Model file for the job. Use its own axes, mm. A direction names the side the tool comes from. Give positions to 0.01 mm unless a question says otherwise; leave off trailing zeros. Write each loop counter-clockwise with the first axis right and the second up, starting at its lowest first coordinate (ties: lowest second). Pieces come first, ordered by that corner, then holes. Notation, with made-up numbers: (77, 40) - (87, 40) arc R4 cw to (87, 47) - close; hole circle Ø5 at (-8, -29.75). An arc over 180 degrees is marked (long way). One line per item, written item: value. Start each with the question number.
(1) Cut at C-C, the plane y = 2.15. State how many separate pieces and enclosed holes the cut face has, and give its area (3 significant figures).
(2) Cut at A-A, the plane x = -10.5. List the corners of the cut face in (y, z).
(3) Cut at B-B, the plane z = -15. List the corners of the cut face in (x, y) (3 decimals), and give its area (3 significant figures).
(4) Probe L1, parallel to Z at x = 30, y = 1.95; L2, parallel to X at y = 2.25, z = 0 (3 decimals); L3, parallel to Z at x = -69, y = 3. List the from-to ranges inside material, lowest first.
(5) Drop flat-ended pins along their axis: P1, Ø2.5, axis at y = 3, z = -113.5, coming from the -X side; P2, Ø2.5, axis at x = 84.63, z = 48.25, coming from the +Y side. Give the stop position or say it passes through.
(6) 3-axis set-ups, long thin cutter, end or side, ignore diameter. For faces 1 (the face through (-19.95, 2.58, 82.46)), 2 (the face through (-119.76, 2.58, 119.36)): which of +Z, -Z, +X, -X, +Y, -Y reach the whole face in a straight line?
(7) Mould opens along Z. For faces 3 (the face through (54.03, 2.58, -94.58)), 4 (the face through (-119.76, 2.58, -119.36)), 5 (the face through (119.36, 2.58, 119.76)) say: pulls with the +Z half, pulls with the -Z half, needs draft (parallel to the pull), parting line crosses it, or undercut.
from build123d import *

# Parameters (mm, degrees)
SKETCH1_W               = 254
SKETCH1_H               = 254
PLATFORM_BASE_DEPTH     = 5.08
SKETCH5_W               = 97.79
SKETCH5_H               = 152.4
CUT_EXTRUDE3_DEPTH      = 180.676950108
SKETCH6_W               = 25.4
SKETCH6_H               = 5.08
CUT_EXTRUDE4_DEPTH      = 180.676950108
CORNER_ROUNDING_R       = 25.4
MIRROR6_COPY_1_SKETCH_W = 25.4
MIRROR6_COPY_1_SKETCH_H = 5.08
MIRROR6_COPY_1_DEPTH    = 180.676950108
SKETCH7_R               = 3.175
CUT_EXTRUDE5_DEPTH      = 180.676950108
SKETCH11_W              = 12.7
SKETCH11_H              = 5.08
CUT_EXTRUDE8_DEPTH      = 180.676950108
SKETCH12_W              = 19.05
SKETCH12_H              = 5.08
CUT_EXTRUDE10_DEPTH     = 16.51
SKETCH14_W              = 152.4
SKETCH14_H              = 8.030698274
CUT_EXTRUDE12_DEPTH     = 19.05
SKETCH16_W              = 76.2
SKETCH16_H              = 5.08
CUT_EXTRUDE14_DEPTH     = 44.45
CUT_EXTRUDE16_DEPTH     = 180.676950108
CUT_EXTRUDE18_DEPTH     = 180.676950108
CUT_EXTRUDE19_DEPTH     = 180.676950108
CUT_EXTRUDE20_DEPTH     = 180.676950108
SKETCH27_W              = 10.16
SKETCH27_H              = 5.08
BOSS_EXTRUDE1_DEPTH     = 177.8
SKETCH28_R              = 1.6
CUT_EXTRUDE22_DEPTH     = 180.676950108
SKETCH29_R              = 1.651
CUT_EXTRUDE23_DEPTH     = 180.676950108
SKETCH30_R              = 1.651
CUT_EXTRUDE24_DEPTH     = 180.676950108
SKETCH32_R              = 1.651
CUT_EXTRUDE26_DEPTH     = 180.676950108


with BuildPart() as part:
    # Sketch1 → Platform-Base (new body)
    with BuildSketch(Plane(origin=(0, 0, 0), x_dir=(1, 0, 0), z_dir=(0, 1, 0))):
        Rectangle(SKETCH1_W, SKETCH1_H)
    extrude(amount=PLATFORM_BASE_DEPTH)

    # Sketch5 → Cut-Extrude3 (cut, through all)
    with BuildSketch(Plane(origin=(0, 5.08, 0), x_dir=(1, 0, 0), z_dir=(0, 1, 0))):
        Rectangle(SKETCH5_W, SKETCH5_H)
    extrude(amount=-CUT_EXTRUDE3_DEPTH, mode=Mode.SUBTRACT)

    # Sketch6 → Cut-Extrude4 (cut, through all)
    with BuildSketch(Plane(origin=(0, 5.08, 0), x_dir=(1, 0, 0), z_dir=(0, 1, 0))):
        with Locations((38.1, -114.3)):
            Rectangle(SKETCH6_W, SKETCH6_H)
    cut_extrude4 = extrude(amount=-CUT_EXTRUDE4_DEPTH, mode=Mode.SUBTRACT)

    # Mirror4: Cut-Extrude4 across plane
    add(cut_extrude4.mirror(Plane.XY), mode=Mode.SUBTRACT)

    # Corner-Rounding
    corner_rounding_edges = [part.edges().sort_by_distance(p)[0] for p in [
        (127, 2.54, 127),
        (-127, 2.54, 127),
        (-127, 2.54, -127),
        (127, 2.54, -127),
    ]]
    fillet(corner_rounding_edges, radius=CORNER_ROUNDING_R)

    # Mirror6: Cut-Extrude4 across plane
    add(cut_extrude4.mirror(Plane.ZY), mode=Mode.SUBTRACT)

    # Mirror6 copy 1 sketch → Mirror6 copy 1 (cut, through all)
    with BuildSketch(Plane(origin=(0, 5.08, 0), x_dir=(-1, 0, 0), z_dir=(0, 1, 0))):
        with Locations((38.1, -114.3)):
            Rectangle(MIRROR6_COPY_1_SKETCH_W, MIRROR6_COPY_1_SKETCH_H)
    extrude(amount=-MIRROR6_COPY_1_DEPTH, mode=Mode.SUBTRACT)

    # Sketch7 → Cut-Extrude5 (cut, through all)
    with BuildSketch(Plane(origin=(0, 5.08, 0), x_dir=(1, 0, 0), z_dir=(0, 1, 0))):
        with Locations(Location((116.84, 0, 0), (0, 0, 270))):
            Circle(SKETCH7_R)
    cut_extrude5 = extrude(amount=-CUT_EXTRUDE5_DEPTH, mode=Mode.SUBTRACT)

    # Mirror7: Cut-Extrude5 across plane
    add(cut_extrude5.mirror(Plane.ZY), mode=Mode.SUBTRACT)

    # Sketch11 → Cut-Extrude8 (cut, through all)
    with BuildSketch(Plane(origin=(0, 5.08, 0), x_dir=(1, 0, 0), z_dir=(0, 1, 0))):
        with Locations((90.17, -5.08)):
            Rectangle(SKETCH11_W, SKETCH11_H)
    extrude(amount=-CUT_EXTRUDE8_DEPTH, mode=Mode.SUBTRACT)

    # Sketch12 → Cut-Extrude10 (cut)
    with BuildSketch(Plane(origin=(0, 5.08, 0), x_dir=(1, 0, 0), z_dir=(0, 1, 0))):
        with Locations((-75.565, -54.61)):
            Rectangle(SKETCH12_W, SKETCH12_H)
    extrude(amount=-CUT_EXTRUDE10_DEPTH, mode=Mode.SUBTRACT)

    # Sketch14 → Cut-Extrude12 (cut)
    with BuildSketch(Plane.ZY.offset(-48.895)):
        with Locations((0, 3.604650863)):
            Rectangle(SKETCH14_W, SKETCH14_H)
    extrude(amount=-CUT_EXTRUDE12_DEPTH, mode=Mode.SUBTRACT)

    # Sketch16 → Cut-Extrude14 (cut)
    with BuildSketch(Plane(origin=(-48.895, 0, 0), x_dir=(0, 0, -1), z_dir=(1, 0, 0))):
        with Locations((0, 2.54)):
            Rectangle(SKETCH16_W, SKETCH16_H)
    extrude(amount=-CUT_EXTRUDE14_DEPTH, mode=Mode.SUBTRACT)

    # Sketch18 → Cut-Extrude16 (cut, through all)
    with BuildSketch(Plane(origin=(0, 5.08, 0), x_dir=(1, 0, 0), z_dir=(0, 1, 0))):
        Polygon((-48.895, 76.2), (-26.616832453, 34.380865163), (67.945, 76.2), (50.165, 99.686546388), (-31.115, 99.686546388), align=None)
    extrude(amount=-CUT_EXTRUDE16_DEPTH, mode=Mode.SUBTRACT)

    # Sketch20 → Cut-Extrude18 (cut, through all)
    with BuildSketch(Plane(origin=(0, 5.08, 0), x_dir=(1, 0, 0), z_dir=(0, 1, 0))):
        Polygon((-48.895, 38.1), (-48.895, 50.8), (-61.595, 38.1), align=None)
    extrude(amount=-CUT_EXTRUDE18_DEPTH, mode=Mode.SUBTRACT)

    # Sketch21 → Cut-Extrude19 (cut, through all)
    with BuildSketch(Plane(origin=(0, 5.08, 0), x_dir=(1, 0, 0), z_dir=(0, 1, 0))):
        Polygon((-48.895, -38.1), (-48.895, -44.45), (-55.245, -38.1), align=None)
    extrude(amount=-CUT_EXTRUDE19_DEPTH, mode=Mode.SUBTRACT)

    # Sketch22 → Cut-Extrude20 (cut, through all)
    with BuildSketch(Plane(origin=(0, 5.08, 0), x_dir=(1, 0, 0), z_dir=(0, 1, 0))):
        Polygon((0, -88.9), (16.51, -88.9), (23.293914706, -76.2), (-5.638297494, -47.784601192), (-23.293914706, -76.2), (-16.51, -88.9), align=None)
    extrude(amount=-CUT_EXTRUDE20_DEPTH, mode=Mode.SUBTRACT)

    # Sketch27 → Boss-Extrude1 (add)
    with BuildSketch(Plane(origin=(0, 0, 76.2), x_dir=(-1, 0, 0), z_dir=(0, 0, -1))):
        with Locations((-62.865, 2.54)):
            Rectangle(SKETCH27_W, SKETCH27_H)
    extrude(amount=BOSS_EXTRUDE1_DEPTH)

    # Sketch28 → Cut-Extrude22 (cut, through all)
    with BuildSketch(Plane.XZ):
        with Locations(Location((-62.993507929, 68.100453228, 0), (0, 0, 270))):
            Circle(SKETCH28_R)
        with Locations(Location((-72.599277809, 45.591362065, 0), (0, 0, 270))):
            Circle(SKETCH28_R)
        with Locations(Location((-71.85594825, -47.293928362, 0), (0, 0, 270))):
            Circle(SKETCH28_R)
        with Locations(Location((-62.446970512, -69.88598754, 0), (0, 0, 270))):
            Circle(SKETCH28_R)
        with Locations(Location((60.907666067, -59.104099387, 0), (0, 0, 270))):
            Circle(SKETCH28_R)
        with Locations(Location((83.684609303, -50.151956805, 0), (0, 0, 270))):
            Circle(SKETCH28_R)
        with Locations(Location((84.63204517, 48.251627594, 0), (0, 0, 270))):
            Circle(SKETCH28_R)
        with Locations(Location((61.507720386, 56.263843475, 0), (0, 0, 270))):
            Circle(SKETCH28_R)
    extrude(amount=-CUT_EXTRUDE22_DEPTH, mode=Mode.SUBTRACT)

    # Sketch29 → Cut-Extrude23 (cut, through all)
    with BuildSketch(Plane(origin=(0, 5.08, 0), x_dir=(1, 0, 0), z_dir=(0, 1, 0))):
        with Locations(Location((-27.25, -123.93, 0), (0, 0, 270))):
            Circle(SKETCH29_R)
        with Locations(Location((-27.25, -89.43, 0), (0, 0, 270))):
            Circle(SKETCH29_R)
        with Locations(Location((27.25, -89.43, 0), (0, 0, 270))):
            Circle(SKETCH29_R)
        with Locations(Location((27.25, -123.93, 0), (0, 0, 270))):
            Circle(SKETCH29_R)
    extrude(amount=-CUT_EXTRUDE23_DEPTH, mode=Mode.SUBTRACT)

    # Sketch30 → Cut-Extrude24 (cut, through all)
    with BuildSketch(Plane(origin=(0, 5.08, 0), x_dir=(1, 0, 0), z_dir=(0, 1, 0))):
        with Locations(Location((101.6, -124.74, 0), (0, 0, 270))):
            Circle(SKETCH30_R)
        with Locations(Location((35.6, -124.74, 0), (0, 0, 270))):
            Circle(SKETCH30_R)
        with Locations(Location((35.6, -78.74, 0), (0, 0, 270))):
            Circle(SKETCH30_R)
        with Locations(Location((101.6, -78.74, 0), (0, 0, 270))):
            Circle(SKETCH30_R)
    extrude(amount=-CUT_EXTRUDE24_DEPTH, mode=Mode.SUBTRACT)

    # Sketch32 → Cut-Extrude26 (cut, through all)
    with BuildSketch(Plane(origin=(0, 5.08, 0), x_dir=(1, 0, 0), z_dir=(0, 1, 0))):
        with Locations(Location((65.76, 35.6, 0), (0, 0, 270))):
            Circle(SKETCH32_R)
        with Locations(Location((111.76, 35.6, 0), (0, 0, 270))):
            Circle(SKETCH32_R)
        with Locations(Location((111.76, 101.6, 0), (0, 0, 270))):
            Circle(SKETCH32_R)
        with Locations(Location((65.76, 101.6, 0), (0, 0, 270))):
            Circle(SKETCH32_R)
    extrude(amount=-CUT_EXTRUDE26_DEPTH, mode=Mode.SUBTRACT)


solid = part.part
Answers follow:
1. separate pieces: 1
1. enclosed holes: 29
1. area: 40,500 mm²
2. outline: (0, -127) - (5.08, -127) - (5.08, -99.69) - (0, -99.69) - close; (0, 88.9) - (5.08, 88.9) - (5.08, 127) - (0, 127) - close
3. outline: (-127, 0) - (-93.345, 0) - (-93.345, 5.08) - (-127, 5.08) - close; (57.785, 0) - (127, 0) - (127, 5.08) - (57.785, 5.08) - close
3. area: 523 mm²
4. L1: z = -127 to -116.84, -111.76 to -99.69, 76.2 to 111.76, 116.84 to 127
4. L2: x = -127 to -120.015, -113.665 to -93.345, 57.785 to 113.665, 120.015 to 127
4. L3: z = -127 to -38.1, 38.1 to 52.07, 57.15 to 127
5. P1: stops at x = -124.66
5. P2: passes through
6. face 1: +Y, -Y
6. face 2: +Z, -X, +Y, -Y
7. face 3: undercut
7. face 4: pulls with the -Z half
7. face 5: pulls with the +Z half
